from build123d import *

# Parameters (mm, degrees)
SKETCH1_W           = 45
SKETCH1_H           = 25
BOSS_EXTRUDE1_DEPTH = 2.5
SKETCH2_W           = 45
SKETCH2_H           = 25
SKETCH2_W_2         = 40
SKETCH2_H_2         = 20
BOSS_EXTRUDE2_DEPTH = 17.5
CUT_EXTRUDE1_DEPTH  = 46


with BuildPart() as part:
    # Sketch1 → Boss-Extrude1 (new body)
    with BuildSketch(Plane(origin=(0, 0, 0), x_dir=(1, 0, 0), z_dir=(0, 1, 0))):
        Rectangle(SKETCH1_W, SKETCH1_H)
    extrude(amount=BOSS_EXTRUDE1_DEPTH)

    # Sketch2 → Boss-Extrude2 (add)
    with BuildSketch(Plane(origin=(0, 2.5, 0), x_dir=(1, 0, 0), z_dir=(0, 1, 0))):
        Rectangle(SKETCH2_W, SKETCH2_H)
        Rectangle(SKETCH2_W_2, SKETCH2_H_2, mode=Mode.SUBTRACT)
    extrude(amount=BOSS_EXTRUDE2_DEPTH)

    # Sketch3 → Cut-Extrude1 (cut, through all)
    with BuildSketch(Plane(origin=(22.5, 0, 0), x_dir=(0, 0, -1), z_dir=(1, 0, 0))):
        with BuildLine():
            Line((-4.25, 12), (-4.25, 20))
            Line((-4.25, 20), (4.25, 20))
            Line((4.25, 20), (4.25, 12))
            ThreePointArc((4.25, 12), (0, 7.75), (-4.25, 12))
        make_face()
    extrude(amount=-CUT_EXTRUDE1_DEPTH, mode=Mode.SUBTRACT)


solid = part.part
Here's how the part is built. I have some questions about the finished solid (model axes, mm). A direction names the side the tool comes from. Round coordinates to 2 decimals unless told otherwise and drop trailing zeros. Write each loop counter-clockwise with the first axis right and the second up, starting at its lowest first coordinate (ties: lowest second). Pieces come first, ordered by that corner, then holes.
1. For faces 1 (the flat face through (22.5, 7.6, 0.2)), 2 (the flat face through (-20, 7, 0)), 3 (the flat face through (-21, 16, 4.25)), which set-ups out of +Z, -Z, +X, -X, +Y, -Y let a thin tool reach every point of the face, with its end or its side?
2. Suppose I cut it at D-D (x = -19.5). List the corners of the cut face in (y, z) for me, and give its area (3 significant figures).
3. Suppose I cut it at C-C (z = 0). List the corners of the cut face in (x, y) for me.
4. I need wall thicknesses on L1, parallel to X at y = 16.5, z = -9.75; L2, parallel to Z at x = 7, y = 5.5; L3, parallel to Y at x = -16.5, z = -4.5. Which ranges of each line are inside material? Lowest first, please.
5. Suppose I cut it at B-B (y = 3.5). List the corners of the cut face in (x, z) for me.
6. Will this pin go through, and if not, where does the flat tip stop? pin 1 Ø1.5 at (x, z) = (12.5, -7) entering from +Y.
7. If we mould it in two halves opening along Z, with no side actions, what happens to faces 4 (the flat face through (-22.5, 7.6, 0.2)), 5 (the flat face through (0, 11, -10)), 6 (the flat face through (0, 10, 12.5))? For each: released by +Z, released by -Z, zero draft, split by the parting line, or undercut.
8. Suppose I cut it at A-A (y = 8.25). List the corners of the cut face in (x, z) for me, and give its area (3 significant figures).
Answer sheet:
1. face 1: +Z, -Z, +X, +Y, -Y
1. face 2: +Y
1. face 3: +X, -X, +Y
2. outline: (0, -12.5) - (20, -12.5) - (20, -10) - (2.5, -10) - (2.5, 10) - (20, 10) - (20, 12.5) - (0, 12.5) - close
2. area: 150 mm2
3. outline: (-22.5, 0) - (22.5, 0) - (22.5, 7.75) - (20, 7.75) - (20, 2.5) - (-20, 2.5) - (-20, 7.75) - (-22.5, 7.75) - close
4. L1: x = -22.5 to -20, 20 to 22.5
4. L2: z = -12.5 to -10, 10 to 12.5
4. L3: y = 0 to 2.5
5. outline: (-22.5, -12.5) - (22.5, -12.5) - (22.5, 12.5) - (-22.5, 12.5) - close; hole (-20, -10) - (20, -10) - (20, 10) - (-20, 10) - close
6. pin 1: stops at y = 2.5
7. face 4: zero draft
7. face 5: undercut
7. face 6: released by +Z
8. outline: (-22.5, -12.5) - (22.5, -12.5) - (22.5, -2) - (20, -2) - (20, -10) - (-20, -10) - (-20, -2) - (-22.5, -2) - close; (-22.5, 2) - (-20, 2) - (-20, 10) - (20, 10) - (20, 2) - (22.5, 2) - (22.5, 12.5) - (-22.5, 12.5) - close
8. area: 305 mm2
